The model under review builds one solid part; all positions refer to its coordinate system, in mm. Face numbers are marked on the shaded views. Round coordinates to 2 decimals unless told otherwise and drop trailing zeros. Loops run counter-clockwise (first coordinate to the right, second up) from the corner with the lowest first, then second, coordinate; pieces in that order, holes last. Notation, with made-up numbers: M 36,0.5 L 95,0.5 A27 ccw 95,16.5 Z; hole C 58.25,-7.75 d6. An arc over 180 degrees is marked long. Return JSON: item names as keys, results as strings. Group by question number.
Q1. To check wall thickness, follow line 1 along X through (y, z) = (50, -0.25); line 2 along X through (y, z) = (66, -3); line 3 along Y through (x, z) = (124, -2). State the ranges of each line that lie inside material, in increasing order.
Q2. Consider section B-B (x = 124). State the section outline as (y, z) points, and give its area (3 significant figures).
Q3. Clearance check with flat-ended pins moving along their axes: pin 1 Ø5 at (y, z) = (106.5, -0.5) entering from +X; pin 2 Ø1.5 at (x, z) = (157, 0.5) entering from -Y. State where each tip first meets the part, or that it passes through.
Q4. Consider section C-C (y = 93.5). State the section outline as (x, z) points.
Q5. Draft analysis for pull direction Y (two halves, no side actions). For the marked faces 1 and 2, state which applies: pulls with the +Y half, pulls with the -Y half, needs draft (parallel to the pull), parting line crosses it, or undercut.
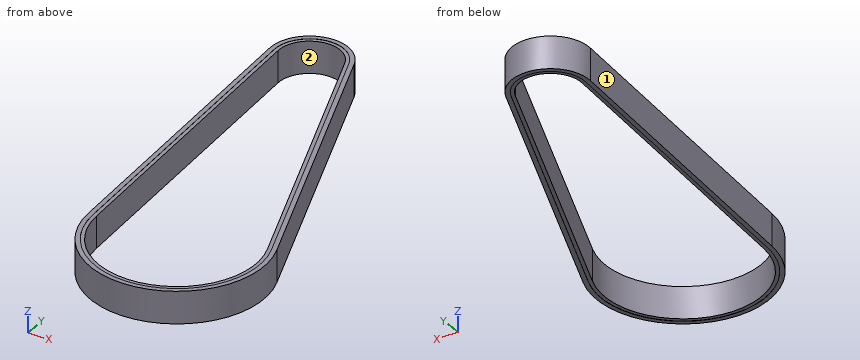
Autodesk Inventor part; units mm, degrees
ref_plane "YZ Plane" through (0, 0, 0) normal (1, 0, 0) x (0, 1, 0)
ref_plane "XZ Plane" through (0, 0, 0) normal (0, 1, 0) x (-1, 0, 0)
ref_plane "XY Plane" through (0, 0, 0) normal (0, 0, 1) x (1, 0, 0)
sketch "Main Outline" plane through (0, 0, 0) normal (0, 0, 1) x (1, 0, 0)
  line L0 (0, 0) -> (304.8, 0) construction
  line L1 (304.8, 0) -> (304.8, 50.8) construction
  line L2 (304.8, 50.8) -> (0, 50.8) construction
  line L3 (0, 50.8) -> (0, 0) construction
  line L4 (0, 50.8) -> (0, 53.34) construction
  line L5 (0, 53.34) -> (304.8, 53.34) construction
  line L6 (304.8, 53.34) -> (304.8, 50.8) construction
  circle A0 centre (152.4, 23.8125) radius 17.4625 construction
  line L7 (152.4, 23.8125) -> (152.4, 0) construction
  circle A1 centre (152.4, 23.8125) radius 27.94 construction
  circle A2 centre (152.4, 23.8125) radius 21.59 construction
  line L8 (152.4, 23.8125) -> (144.1569, 60.2292) construction
  circle A3 centre (144.1569, 60.2292) radius 15.24 construction
  circle A4 centre (144.1569, 60.2292) radius 8.89 construction
  circle A5 centre (144.1569, 60.2292) radius 14.2875 construction
  arc A6 (163.8162, 72.0089) -> (128.198, 43.7805) centre (144.1569, 60.2292) ccw construction
  circle A7 centre (98.8106, 85.598) radius 32.258 construction
  circle A8 centre (124.5097, 147.0273) radius 32.258 construction
  circle A9 centre (174.158, 102.6533) radius 32.258 construction
  circle A10 centre (144.1569, 60.2292) radius 11.1125 construction
  circle A11 centre (152.4, 23.8125) radius 49.53 construction
  line L9 (144.1569, 60.2292) -> (124.5097, 147.0273) construction
  line L10 (144.1569, 60.2292) -> (98.8106, 85.598) construction
  line L11 (98.8106, 85.598) -> (174.158, 102.6533) construction
  line L12 (174.158, 102.6533) -> (144.1569, 60.2292) construction
  circle A12 centre (98.8106, 85.598) radius 9.5493 construction
  arc A13 (172.0498, 111.9669) -> (183.1109, 99.3313) centre (174.158, 102.6533) ccw construction
  circle A14 centre (124.5097, 147.0273) radius 9.5493 construction
  line L13 (96.7024, 94.9117) -> (172.0498, 111.9669) construction
  line L14 (183.1109, 99.3313) -> (165.6438, 52.2565) construction
  line L15 (92.161, 78.7444) -> (128.198, 43.7805) construction
  line L16 (172.0498, 111.9669) -> (174.158, 102.6533) construction
  line L17 (174.158, 102.6533) -> (183.1109, 99.3313) construction
  arc A15 (183.1109, 99.3313) -> (172.0498, 111.9669) centre (174.158, 102.6533) ccw construction
  arc A16 (165.6438, 52.2565) -> (163.8162, 72.0089) centre (144.1569, 60.2292) ccw construction
  arc A17 (128.198, 43.7805) -> (165.6438, 52.2565) centre (144.1569, 60.2292) ccw construction
  circle A18 centre (124.4396, 147.337) radius 32.258 construction
  circle A19 centre (124.3695, 147.6466) radius 32.258 construction
  circle A20 centre (124.2994, 147.9563) radius 32.258 construction
  line L18 (124.5097, 147.0273) -> (124.2994, 147.9563) construction
  circle A21 centre (124.5798, 146.7176) radius 32.258 construction
  circle A22 centre (117.4622, 43.2997) radius 9.525 construction
  circle A23 centre (175.54, 56.4459) radius 9.525 construction
  line L19 (152.4, 23.8125) -> (117.4622, 43.2997) construction
  line L20 (152.4, 23.8125) -> (175.54, 56.4459) construction
  line L21 (117.4622, 43.2997) -> (98.8106, 85.598) construction
  line L22 (175.54, 56.4459) -> (174.158, 102.6533) construction
  circle A24 centre (133.7342, 106.2753) radius 7.9375 construction
  line L23 (133.401, 150.5107) -> (165.496, 68.5894) construction
  circle A25 centre (152.4, 23.8125) radius 29.845 construction
  line L24 (114.985, 146.3422) -> (121.2977, 58.5849) construction
  circle A26 centre (99.0876, 85.443) radius 32.258 construction
  circle A27 centre (97.9793, 86.063) radius 32.258 construction
  line L25 (97.9793, 86.063) -> (98.8106, 85.598) construction
  circle A28 centre (98.2564, 85.908) radius 32.258 construction
  circle A29 centre (98.5335, 85.753) radius 32.258 construction
  circle A30 centre (152.4, 23.8125) radius 29.845 construction
  circle A31 centre (122.555, 23.8125) radius 6.35 construction
  circle A32 centre (179.3358, 36.6651) radius 6.35 construction
  line L26 (122.555, 23.8125) -> (152.4, 23.8125) construction
  line L27 (152.4, 23.8125) -> (182.245, 23.8125) construction
  circle A33 centre (182.245, 23.8125) radius 6.35 construction
  circle A34 centre (125.4642, 10.9599) radius 6.35 construction
  circle A35 centre (150.1885, 33.5827) radius 39.8623 construction
  line L28 (72.8944, 65.7819) -> (119.1902, 8.5205) construction
  circle A36 centre (174.708, 103.431) radius 32.258 construction
  line L29 (174.158, 102.6533) -> (174.708, 103.431) construction
  circle A37 centre (174.5246, 103.1717) radius 32.258 construction
  circle A38 centre (174.3413, 102.9125) radius 32.258 construction
  circle A39 centre (173.9747, 102.394) radius 32.258 construction
  line L30 (188.958, 24.3128) -> (206.0816, 95.9295) construction
  circle A40 centre (133.7342, 106.2753) radius 8.1693 construction
  arc A41 (85.4541, 115.7901) -> (94.2274, 135.7949) centre (79.2901, 130.4196) ccw construction
  arc A42 (156.6774, 149.9308) -> (173.2104, 135.6542) centre (172.4734, 151.5121) ccw construction
  line L31 (124.2994, 147.9563) -> (124.8602, 145.479) construction
  line L32 (114.3901, 145.7133) -> (114.9509, 143.236) construction
  line L33 (134.7695, 147.722) -> (134.2088, 150.1993) construction
  arc A43 (134.2088, 150.1993) -> (114.3901, 145.7133) centre (124.2994, 147.9563) ccw construction
  arc A44 (114.9509, 143.236) -> (134.7695, 147.722) centre (124.8602, 145.479) ccw construction
  line L34 (174.708, 103.431) -> (173.2414, 101.3571) construction
  line L35 (166.4126, 109.2972) -> (164.9461, 107.2234) construction
  line L36 (181.5368, 95.4909) -> (183.0033, 97.5647) construction
  arc A45 (183.0033, 97.5647) -> (166.4126, 109.2972) centre (174.708, 103.431) ccw construction
  arc A46 (164.9461, 107.2234) -> (181.5368, 95.4909) centre (173.2414, 101.3571) ccw construction
  line L37 (97.9793, 86.063) -> (100.196, 84.8229) construction
  line L38 (93.0188, 77.1963) -> (95.2355, 75.9562) construction
  line L39 (105.1564, 93.6897) -> (102.9398, 94.9298) construction
  arc A47 (102.9398, 94.9298) -> (93.0188, 77.1963) centre (97.9793, 86.063) ccw construction
  arc A48 (95.2355, 75.9562) -> (105.1564, 93.6897) centre (100.196, 84.8229) ccw construction
  circle A49 centre (117.4622, 43.2997) radius 3.9687 construction
  circle A50 centre (175.54, 56.4459) radius 3.9687 construction
  line L40 (152.4, 23.8125) -> (158.9889, -5.2961) construction
  arc A51 (89.3511, 54.6895) -> (85.9237, 49.6664) centre (88.3927, 51.6626) ccw construction
  arc A52 (201.2624, 75.7739) -> (196.006, 78.8314) centre (198.1744, 76.5122) ccw construction
  circle A53 centre (152.4, 23.8125) radius 14.224 construction
  circle A54 centre (133.7342, 106.2753) radius 3.9687 construction
  circle A55 centre (156.886, 3.9939) radius 6.35 construction
  circle A56 centre (156.886, 3.9939) radius 2.0828 construction
  circle A57 centre (152.4, 23.8125) radius 20.32 construction
  line L41 (132.9935, 29.8368) -> (152.4, 23.8125) construction
  line L42 (152.4, 23.8125) -> (167.3204, 37.6068) construction
  circle A58 centre (167.3204, 37.6068) radius 2.0828 construction
  circle A59 centre (167.3204, 37.6068) radius 3.9687 construction
  circle A60 centre (132.9935, 29.8368) radius 2.0828 construction
  circle A61 centre (132.9935, 29.8368) radius 3.9688 construction
  point P0 (173.9747, 102.394)
  point P1 (99.0876, 85.443)
  dimension "d18" = 99.06
  dimension "d58" = 64.516
  dimension "d86" = 64.516
  dimension "d0" = 304.8
  dimension "d1" = 50.8
  dimension "d2" = 2.54
  dimension "d3" = 34.925
  dimension "d4" = 23.8125
  dimension "d5" = 152.4
  dimension "d6" = 55.88
  dimension "d7" = 43.18
  dimension "d8" = 37.338
  dimension "d10" = 30.48
  dimension "d11" = 17.78
  dimension "d12" = 28.575
  dimension "d13" = 45.8366
  dimension "d14" = 64.516
  dimension "d15" = 64.516
  dimension "d16" = 64.516
  dimension "d17" = 22.225
  dimension "d19" = 51.9602
  dimension "d20" = 88.9939
  dimension "d21" = 19.0986
  dimension "d22" = 19.0986
  dimension "d23" = 19.0986
  dimension "d30" = 123.112
  dimension "d40" = 64.516
  dimension "d41" = 64.516
  dimension "d42" = 64.516
  dimension "d43" = 0.9525
  dimension "d44" = 0.3175
  dimension "d45" = 0.635
  dimension "d46" = 64.516
  dimension "d47" = 0.3175
  dimension "d48" = 19.05
  dimension "d49" = 19.05
  dimension "d50" = 40.005
  dimension "d51" = 40.005
  dimension "d52" = 46.228
  dimension "d54" = 46.228
  dimension "d55" = 15.875
  dimension "d56" = 41.4655
  dimension "d57" = 59.69
  dimension "d59" = 64.516
  dimension "d60" = 64.516
  dimension "d61" = 64.516
  dimension "d62" = 0.3175
  dimension "d63" = 0.3175
  dimension "d64" = 0.635
  dimension "d65" = 0.9525
  dimension "d73" = 12.7
  dimension "d74" = 12.7
  dimension "d76" = 59.69
  dimension "d78" = 12.7
  dimension "d79" = 12.7
  dimension "d80" = 64.516
  dimension "d81" = 0.9525
  dimension "d82" = 64.516
  dimension "d83" = 64.516
  dimension "d84" = 0.3175
  dimension "d85" = 0.635
  dimension "d88" = 0.3175
  dimension "d89" = 31.75
  dimension "d90" = 31.75
  dimension "d94" = 1.5875
  dimension "d95" = 20.32
  dimension "d96" = 1.5875
sketch "Upper CIM C-C Check" plane through (0, 0, 0) normal (0, 0, 1) x (1, 0, 0)
  arc A0 (3.4429, -22.6582) -> (3.4429, 22.6582) centre (0, 0) ccw construction
  arc A1 (90.4285, 9.4409) -> (90.4285, -9.4409) centre (88.9939, 0) ccw construction
  line L0 (88.9939, 0) -> (0, 0) construction
  line L1 (90.4285, 9.4409) -> (3.4429, 22.6582)
  line L2 (3.4429, -22.6582) -> (90.4285, -9.4409)
  arc A2 (90.4285, -9.4409) -> (90.4285, 9.4409) centre (88.9939, 0) ccw
  arc A3 (3.4429, 22.6582) -> (3.4429, -22.6582) centre (0, 0) ccw
  dimension "d24" = 45.8366
  dimension "d25" = 19.0986
  dimension "d26" = 78.9119
  dimension "d27" = 87.984
  dimension "d28" = 27.12
  dimension "d29" = 88.9939
sketch "Sketch3" plane through (0, 0, 0) normal (0, 0, 1) x (1, 0, 0)
  line L0 (114.985, 146.3422) -> (121.2977, 58.5849)
  line L1 (133.401, 150.5107) -> (165.496, 68.5894)
  arc A0 (133.401, 150.5107) -> (114.985, 146.3422) centre (124.5097, 147.0273) ccw
  arc A1 (121.2977, 58.5849) -> (165.496, 68.5894) centre (144.1569, 60.2292) ccw
  line L2 (164.55, 68.2188) -> (132.455, 150.1401)
  arc A2 (132.455, 150.1401) -> (115.9984, 146.4151) centre (124.5097, 147.0273) ccw
  line L3 (115.9984, 146.4151) -> (122.311, 58.6578)
  arc A3 (122.311, 58.6578) -> (164.55, 68.2188) centre (144.1569, 60.2292) ccw
  line L4 (166.6785, 69.0527) -> (134.5835, 150.974)
  arc A4 (134.5835, 150.974) -> (113.7183, 146.2511) centre (124.5097, 147.0273) ccw
  line L5 (113.7183, 146.2511) -> (120.0309, 58.4938)
  arc A5 (120.0309, 58.4938) -> (166.6785, 69.0527) centre (144.1569, 60.2292) ccw
  point P0 (0, 0)
  dimension "d115" = 1.27
  dimension "d116" = 1.016
extrude "Extrusion1" add sketch "Sketch3" along normal blind 4.5 contours A5 L5 A4 L4
extrude "Extrusion2" add sketch "Sketch3" along normal blind 4.45 contours A0 L1 A1 L0
mirror "Mirror1" about plane through (136.0096, 96.2228, 0) normal (0, 0, -1)
equation "\"d3\" = r10"
equation "\"d6\" = g44"
equation "\"d7\" = g34"
equation "\"d10\" = g24"
equation "\"d11\" = g14"
equation "\"d12\" = r8"
equation "\"d13\" = p48"
equation "\"d14\" = cim"
equation "\"d15\" = cim"
equation "\"d16\" = cim"
equation "\"d17\" = r6"
equation "\"d21\" = p20"
equation "\"d22\" = p20"
equation "\"d23\" = p20"
equation "\"d24\" = p48"
equation "\"d25\" = p20"
equation "\"d29\" = d20"
equation "\"g14\" = 17.78"
equation "\"g24\" = 30.48"
equation "\"g34\" = 43.18"
equation "\"g44\" = 55.88"
equation "\"p20\" = 19.09859"
equation "\"p48\" = 45.83662"
equation "\"r10\" = 34.925"
equation "\"r9\" = 31.75"
equation "\"r8\" = 28.575"
equation "\"r7\" = 25.4"
equation "\"r6\" = 22.225"
equation "\"r5\" = 19.05"
equation "\"r4\" = 15.875"
equation "\"r3\" = 12.7"
equation "\"cim\" = 64.516"
equation "\"act\" = 28.448"
equation "\"actL\" = 23.749"
equation "\"UpperCimCCCheck\" = 2 * d27 + d26 + d28"
equation "\"LowerBeltPathCCCheck\" = 267"
properties material "Rubber"
Values:
{
 "1": {"line 1": "x = 122.24 to 124.79, 163.52 to 166.08", "line 2": "x = 119.49 to 121.78, 165.29 to 167.65", "line 3": "y = 46.86 to 51.66, 155.55 to 157.83"},
 "2": {"outline": "M 46.86,-4.5 L 49.32,-4.5 L 49.32,-4.45 L 51.66,-4.45 L 51.66,4.45 L 49.32,4.45 L 49.32,4.5 L 46.86,4.5 Z; M 155.55,-4.45 L 156.56,-4.45 L 156.56,-4.5 L 157.83,-4.5 L 157.83,4.5 L 156.56,4.5 L 156.56,4.45 L 155.55,4.45 Z", "area": "63.5 mm2"},
 "3": {"pin 1": "stops at x = 152.99", "pin 2": "stops at y = 39.28"},
 "4": {"outline": "M 117.51,-4.5 L 118.79,-4.5 L 118.79,-4.45 L 119.8,-4.45 L 119.8,4.45 L 118.79,4.45 L 118.79,4.5 L 117.51,4.5 Z; M 154.65,-4.45 L 155.74,-4.45 L 155.74,-4.5 L 157.1,-4.5 L 157.1,4.5 L 155.74,4.5 L 155.74,4.45 L 154.65,4.45 Z"},
 "5": {"face 1": "pulls with the -Y half", "face 2": "undercut"}
}
